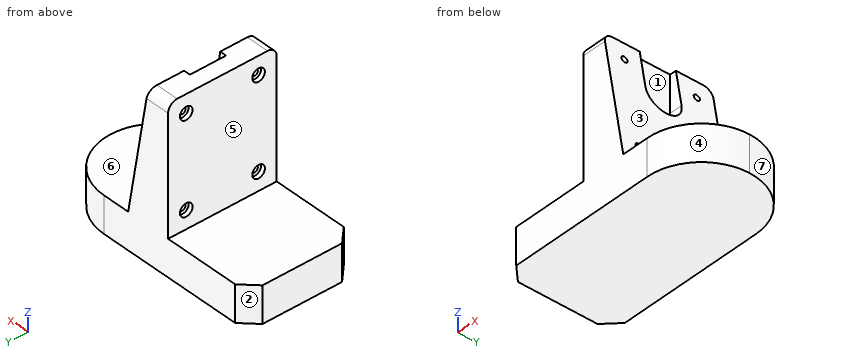
from build123d import *

# Parameters (mm, degrees)
F0_W           = 120
F0_H           = 60
F1_DEPTH       = 90
F2_W           = 50
F2_H           = 70
F2_W_2         = 45
F3_DEPTH       = 60.001
F4_R           = 29.99999
F5_SIZE        = 8
F7_D           = 3.4
F7_CBORE_D     = 7
F7_CBORE_DEPTH = 2.4
F9_DEPTH       = 16
F11_DEPTH      = 60.001
F12_R          = 5


# Not quite as in the source:
# - a fillet or chamfer is up to 0.001 mm smaller than in the source, because OpenCascade refuses the exact size


with BuildPart() as f1:
    # F0 (on Top) → F1 (new body)
    with BuildSketch(Plane.XY):
        with Locations((60, 30)):
            Rectangle(F0_W, F0_H)
    extrude(amount=F1_DEPTH)

    # F2 (on face) → F3 (cut, through all)
    with BuildSketch(Plane.XZ):
        with Locations((25, 55)):
            Rectangle(F2_W, F2_H)
        with Locations((97.5, 55)):
            Rectangle(F2_W_2, F2_H)
    extrude(amount=-F3_DEPTH, mode=Mode.SUBTRACT)

    # F4 (radius 30 in the source; OpenCascade refuses exactly that, so slightly less here)
    f4_edges = [f1.edges().sort_by_distance(p)[0] for p in [
        (120, 60, 10),
        (120, 0, 10),
    ]]
    fillet(f4_edges, radius=F4_R)

    # F5
    f5_edges = [f1.edges().sort_by_distance(p)[0] for p in [
        (0, 60, 10),
        (0, 0, 10),
    ]]
    chamfer(f5_edges, length=F5_SIZE)

    # F7 (through all)
    with Locations(Plane(origin=(50, 0, 0), x_dir=(0, -1, 0), z_dir=(-1, 0, 0))):
        with Locations((-50, 80), (-10, 80), (-10, 30), (-50, 30)):
            CounterBoreHole(F7_D / 2, F7_CBORE_D / 2, F7_CBORE_DEPTH)

    # F8 (on face) → F9 (cut)
    with BuildSketch(Plane.YZ.offset(75)):
        with BuildLine():
            Line((40, 90), (20, 90))
            Line((20, 90), (20, 70))
            ThreePointArc((20, 70), (30, 80), (40, 70))
            Line((40, 70), (40, 90))
        make_face()
        with BuildLine():
            ThreePointArc((40, 70), (30, 80), (20, 70))
            Line((20, 70), (40, 70))
        make_face()
        with BuildLine():
            Line((40, 70), (20, 70))
            ThreePointArc((20, 70), (30, 60), (40, 70))
        make_face()
    extrude(amount=-F9_DEPTH, mode=Mode.SUBTRACT)

    # F10 (on face) → F11 (cut, through all)
    with BuildSketch(Plane.XZ):
        Polygon((62.6571113504, 90), (75, 20), (75, 90), align=None)
    extrude(amount=-F11_DEPTH, mode=Mode.SUBTRACT)

    # F12
    f12_edges = [f1.edges().sort_by_distance(p)[0] for p in [
        (56.328556, 60, 90),
        (56.328556, 0, 90),
    ]]
    fillet(f12_edges, radius=F12_R)


solid = f1.part
Model file for the job. Use its own axes, mm. Face numbers are marked on the shaded views. A direction names the side the tool comes from. Give positions to 0.01 mm unless a question says otherwise; leave off trailing zeros. Loops run counter-clockwise (first coordinate to the right, second up) from the corner with the lowest first, then second, coordinate; pieces in that order, holes last.
1) Tool access for the marked faces 5, 6 and 7: list every direction of +Z, -Z, +X, -X, +Y, -Y with a clear straight run to the whole face (end or side of a thin tool).
2) Wall check: line 1 (Z direction, x = 51, y = 10); line 2 (Y direction, x = 59.25, z = 30); line 3 (Z direction, x = 55, y = 50). Give the ranges that are in metal, low to high.
3) Pull direction Y, two halves, no side cores. Call the marked faces 1, 2, 3 and 4: +Y half, -Y half, draft (parallel to the pull), parting line (faces both ways), or undercut.
4) Flat gauge pins, fed straight in: pin 1 Ø5.5 at (y, z) = (50.5, 80.5) entering from -X; pin 2 Ø1 at (x, z) = (97.5, 16) entering from -Y; pin 3 Ø4 at (y, z) = (10, 80) entering from +X. Where does each tip first touch, or does it go through?
5) Saw through at C-C (y = 42). Write the cut outline in (x, z), plus the area to 3 significant figures.
6) Saw through at B-B (z = 30). Write the cut outline in (x, y).
7) Saw through at A-A (x = 61). Write the cut outline in (y, z), plus the area to 3 significant figures.
Answer block:
1. face 5: +Z, -X, +Y, -Y
1. face 6: +Z, +X, +Y, -Y
1. face 7: +Z, -Z, +X, +Y
2. line 1: z = 0 to 26.5, 33.5 to 76.5, 83.5 to 90
2. line 2: y = 0 to 8.3, 11.7 to 48.3, 51.7 to 60
2. line 3: z = 0 to 28.3, 31.7 to 78.3, 81.7 to 90
3. face 1: undercut
3. face 2: +Y half
3. face 3: draft
3. face 4: -Y half
4. pin 1: stops at x = 52.4
4. pin 2: stops at y = 0.83
4. pin 3: stops at x = 64.77
5. outline: (0, 0) - (117.5, 0) - (117.5, 20) - (75, 20) - (62.66, 90) - (50, 90) - (50, 20) - (0, 20) - close
5. area: 3,670 mm2
6. outline: (50, 0) - (73.24, 0) - (73.24, 8.3) - (52.4, 8.3) - (52.4, 6.5) - (50, 6.5) - close; (50, 13.5) - (52.4, 13.5) - (52.4, 11.7) - (73.24, 11.7) - (73.24, 48.3) - (52.4, 48.3) - (52.4, 46.5) - (50, 46.5) - close; (50, 53.5) - (52.4, 53.5) - (52.4, 51.7) - (73.24, 51.7) - (73.24, 60) - (50, 60) - close
7. outline: (0, 0) - (60, 0) - (60, 85) arc R5 ccw to (55, 90) - (40, 90) - (40, 70) arc R10 cw to (20, 70) - (20, 90) - (5, 90) arc R5 ccw to (0, 85) - close; hole circle Ø3.4 at (10, 30); hole circle Ø3.4 at (10, 80); hole circle Ø3.4 at (50, 30); hole circle Ø3.4 at (50, 80)
7. area: 4,800 mm2
